Source: CAD feature listing. Evaluate the final solid. Frame: model axes, mm. Round coordinates to 2 decimals unless told otherwise and drop trailing zeros. Loops run counter-clockwise (first coordinate to the right, second up) from the corner with the lowest first, then second, coordinate; pieces in that order, holes last. Notation, with made-up numbers: M 37.5,82.25 L 75.5,82.25 A10 cw 75.5,93.25 Z; hole C 4.25,1.5 d3. An arc over 180 degrees is marked long. Answer as a JSON object with one key per item and string values.
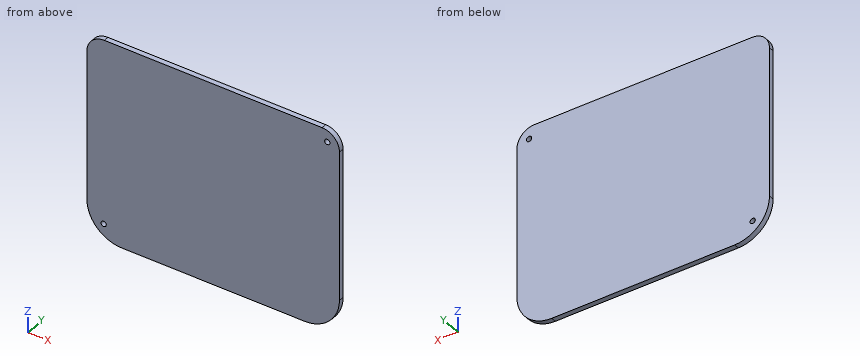
from build123d import *

# Parameters (mm, degrees)
SKETCH1_W           = 145
SKETCH1_H           = 115
BOSS_EXTRUDE1_DEPTH = 3
FILLET1_R           = 10
FILLET2_R           = 20
CUT_EXTRUDE1_REACH  = 5
SKETCH2_R           = 1.5


with BuildPart() as part:
    # Sketch1 → Boss-Extrude1 (new body)
    with BuildSketch(Plane(origin=(0, 0, 0), x_dir=(1, 0, 0), z_dir=(0, 1, 0))):
        Rectangle(SKETCH1_W, SKETCH1_H)
    extrude(amount=BOSS_EXTRUDE1_DEPTH)

    # Fillet1
    fillet1_edges = [part.edges().sort_by_distance(p)[0] for p in [
        (72.5, 1.5, 57.5),
        (-72.5, 1.5, 57.5),
    ]]
    fillet(fillet1_edges, radius=FILLET1_R)

    # Fillet2
    fillet2_edges = [part.edges().sort_by_distance(p)[0] for p in [
        (-72.5, 1.5, -57.5),
        (72.5, 1.5, -57.5),
    ]]
    fillet(fillet2_edges, radius=FILLET2_R)

    # Sketch2 → Cut-Extrude1 (cut, up to next)
    with BuildSketch(Plane.XZ, mode=Mode.PRIVATE) as cut_extrude1_sk1:
        with Locations((65.5, 50.5)):
            Circle(SKETCH2_R)
    cut_extrude1_tool1 = extrude(cut_extrude1_sk1.sketch, amount=-CUT_EXTRUDE1_REACH, mode=Mode.PRIVATE) & part.part
    add(cut_extrude1_tool1.solids().sort_by_distance((65.5, 0, 50.5))[0], mode=Mode.SUBTRACT)
    # Sketch2 → Cut-Extrude1 (cut, up to next)
    with BuildSketch(Plane.XZ, mode=Mode.PRIVATE) as cut_extrude1_sk2:
        with Locations((-62.868103764, -47.867300771)):
            Circle(SKETCH2_R)
    cut_extrude1_tool2 = extrude(cut_extrude1_sk2.sketch, amount=-CUT_EXTRUDE1_REACH, mode=Mode.PRIVATE) & part.part
    add(cut_extrude1_tool2.solids().sort_by_distance((-62.868104, 0, -47.867301))[0], mode=Mode.SUBTRACT)


solid = part.part
Item 1: Section B-B on x = 65.5. Return the cut outline in (y, z), then the cut area to 3 significant figures.
Answer sheet:
{"outline": "M 0,-52.7 L 3,-52.7 L 3,49 L 0,49 Z; M 0,52 L 3,52 L 3,57.04 L 0,57.04 Z", "area": "320 mm²"}
Item 2: Line query: probe 1 along Z at (x, y) = (65.5, 1.8); probe 2 along X at (y, z) = (2.8, -47); probe 3 along Z at (x, y) = (-64, 0.3). Output: solid intervals per line, ascending. Write a range as from..to.
Answer sheet:
{"probe 1": "z = -52.7..49, 52..57.04", "probe 2": "x = -70.1..-64.09, -61.64..70.1", "probe 3": "z = -53.86..-48.85, -46.88..57.39"}
Item 3: Section C-C on z = -44.5. Return the cut outline in (x, y) (3 decimals), then the cut area to 3 significant figures.
Answer sheet:
{"outline": "M -71.235,0 L 71.235,0 L 71.235,3 L -71.235,3 Z", "area": "427 mm²"}
Item 4: Section A-A on z = 50.5. Return the cut outline in (x, y), then the cut area to 3 significant figures.
Answer sheet:
{"outline": "M -72.04,0 L 64,0 L 64,3 L -72.04,3 Z; M 67,0 L 72.04,0 L 72.04,3 L 67,3 Z", "area": "423 mm²"}
Item 5: Contact query for flat-ended pins moving along their axis: pin 1 Ø12 at (x, z) = (24, -40) entering from -Y; pin 2 Ø1.8 at (x, z) = (65.5, 50.5) entering from +Y. Output: stop coordinate, or through.
Answer sheet:
{"pin 1": "stops at y = 0", "pin 2": "passes through"}
